from build123d import *

# Parameters (mm, degrees)
SKETCH1_W           = 17
SKETCH1_H           = 17
BOSS_EXTRUDE1_DEPTH = 120
SKETCH2_W           = 5
SKETCH2_H           = 20
CUT_EXTRUDE1_DEPTH  = 124.288280059
SKETCH3_R           = 3
CUT_EXTRUDE2_DEPTH  = 100
SKETCH4_R           = 2
CUT_EXTRUDE3_DEPTH  = 10


with BuildPart() as part:
    # Sketch1 → Boss-Extrude1 (new body)
    with BuildSketch(Plane(origin=(0, 0, 0), x_dir=(1, 0, 0), z_dir=(0, 1, 0))):
        with BuildLine():
            Line((0.5, 0), (19.5, 0))
            ThreePointArc((19.5, 0), (19.853553391, 0.146446609), (20, 0.5))
            Line((20, 0.5), (20, 19.5))
            ThreePointArc((20, 19.5), (19.853553391, 19.853553391), (19.5, 20))
            Line((19.5, 20), (0.5, 20))
            ThreePointArc((0.5, 20), (0.146446609, 19.853553391), (0, 19.5))
            Line((0, 19.5), (0, 0.5))
            ThreePointArc((0, 0.5), (0.146446609, 0.146446609), (0.5, 0))
        make_face()
        with Locations((10, 10)):
            Rectangle(SKETCH1_W, SKETCH1_H, mode=Mode.SUBTRACT)
    extrude(amount=BOSS_EXTRUDE1_DEPTH)

    # Sketch2 → Cut-Extrude1 (cut, through all)
    with BuildSketch(Plane(origin=(20, 0, 0), x_dir=(0, 0, -1), z_dir=(1, 0, 0))):
        with Locations((17.5, 102)):
            Rectangle(SKETCH2_W, SKETCH2_H)
        with Locations((17.5, 18)):
            Rectangle(SKETCH2_W, SKETCH2_H)
    extrude(amount=-CUT_EXTRUDE1_DEPTH, mode=Mode.SUBTRACT)

    # Sketch3 → Cut-Extrude2 (cut)
    with BuildSketch(Plane.XY):
        with Locations((10, 102)):
            Circle(SKETCH3_R)
        with Locations((10, 18)):
            Circle(SKETCH3_R)
    extrude(amount=-CUT_EXTRUDE2_DEPTH, mode=Mode.SUBTRACT)

    # Sketch4 → Cut-Extrude3 (cut)
    with BuildSketch(Plane.XY):
        with Locations((14.25, 83.15)):
            Circle(SKETCH4_R)
        with Locations(Location((14.25, 36.85, 0), (0, 0, 180))):
            Circle(SKETCH4_R)
    extrude(amount=-CUT_EXTRUDE3_DEPTH, mode=Mode.SUBTRACT)


solid = part.part
The model under review builds one solid part; all positions refer to its coordinate system, in mm. A direction names the side the tool comes from. Give positions to 0.01 mm unless a question says otherwise; leave off trailing zeros. Loops run counter-clockwise (first coordinate to the right, second up) from the corner with the lowest first, then second, coordinate; pieces in that order, holes last. Notation, with made-up numbers: (64, 63.25) -> (95, 63.25) arc R25 ccw to (95, 99.25) -> close; hole circle Ø7 at (52, 12). An arc over 180 degrees is marked (long way). Put each result on its own line as item: value. Start each with the question number.
1. Clearance check with flat-ended pins moving along their axes: P1, Ø3.5, axis at x = 10, y = 18, coming from the -Z side (3 decimals); P2, Ø1.2, axis at x = 19.5, y = 20.5, coming from the -Z side. State where each tip first meets the part, or that it passes through.
2. Wall thickness on probe 1 along Y at (x, z) = (14.25, -0.45); probe 2 along Z at (x, y) = (7, 71); probe 3 along Y at (x, z) = (10, -0.85): over which ranges is each line inside the solid? List them lowest first.
3. We need section C-C on z = -6. State the section outline as (x, y) points.
4. Mouldability with a two-part tool opening along Y and no side actions: class faces 1 (the face through (1, 120, -10)), 2 (the face through (1, 0, -10)), 3 (the face through (18.5, 59, -10)), 4 (the face through (10, 92, -19)) as released by +Y, released by -Y, zero draft, split by the parting line, or undercut.
5. We need section D-D on x = 4. State the section outline as (y, z) points.
6. We need section B-B on y = 53.5. State the section outline as (x, z) points, then the cut area to 3 significant figures.
7. For faces 5 (the face through (13.8, 81.2, -0.7)), 6 (the face through (10, 8, -19)), 7 (the face through (10, 60, -18.5)), 8 (the face through (10, 116, -20)), 9 (the face through (9.35, 99.07, -0.74)), list the 3-axis set-ups (+Z, -Z, +X, -X, +Y, -Y) from which the entire face can be reached by the end or side of a thin tool; tool diameter is ignored.
8. We need section A-A on x = 14.25. State the section outline as (y, z) points.
Determined:
1. P1: through
1. P2: z = -15
2. probe 1: 0 to 34.85, 38.85 to 81.15, 85.15 to 120
2. probe 2: -20 to -18.5, -1.5 to 0
2. probe 3: 0 to 15, 21 to 99, 105 to 120
3. outline: (0, 0) -> (1.5, 0) -> (1.5, 120) -> (0, 120) -> close; (18.5, 0) -> (20, 0) -> (20, 120) -> (18.5, 120) -> close
4. face 1: released by +Y
4. face 2: released by -Y
4. face 3: zero draft
4. face 4: undercut
5. outline: (0, -20) -> (8, -20) -> (8, -18.5) -> (0, -18.5) -> close; (0, -1.5) -> (120, -1.5) -> (120, 0) -> (0, 0) -> close; (28, -20) -> (92, -20) -> (92, -18.5) -> (28, -18.5) -> close; (112, -20) -> (120, -20) -> (120, -18.5) -> (112, -18.5) -> close
6. outline: (0, -19.5) arc R0.5 ccw to (0.5, -20) -> (19.5, -20) arc R0.5 ccw to (20, -19.5) -> (20, -0.5) arc R0.5 ccw to (19.5, 0) -> (0.5, 0) arc R0.5 ccw to (0, -0.5) -> close; hole (1.5, -18.5) -> (18.5, -18.5) -> (18.5, -1.5) -> (1.5, -1.5) -> close
6. area: 111 mm^2
7. face 5: +Z
7. face 6: -Z, +X, -X
7. face 7: +Y, -Y
7. face 8: -Z, +X, -X, +Y, -Y
7. face 9: +Z, -Z
8. outline: (0, -20) -> (8, -20) -> (8, -18.5) -> (0, -18.5) -> close; (0, -1.5) -> (34.85, -1.5) -> (34.85, 0) -> (0, 0) -> close; (28, -20) -> (92, -20) -> (92, -18.5) -> (28, -18.5) -> close; (38.85, -1.5) -> (81.15, -1.5) -> (81.15, 0) -> (38.85, 0) -> close; (85.15, -1.5) -> (120, -1.5) -> (120, 0) -> (85.15, 0) -> close; (112, -20) -> (120, -20) -> (120, -18.5) -> (112, -18.5) -> close
